```python
from build123d import *

# Parameters (mm, degrees)
F0_W     = 33
F0_H     = 70
F0_W_2   = 12.5
F0_H_2   = 29.0257008746
F0_R     = 1.95
F0_H_3   = 10
F1_DEPTH = 10
F2_DEPTH = 28
F3_START = 10
F3_DEPTH = 11
F4_SIZE2 = 8
F4_SIZE  = 2
F5_R     = 4
F6_R     = 5
F7_R     = 2
F8_R     = 2


with BuildPart() as f1:
    # F0 (on Top) → F1 (new body)
    with BuildSketch(Plane.XY):
        with Locations((-48.7103275061, 13.0742679536)):
            Rectangle(F0_W, F0_H)
        with Locations((-48.9603275061, -3.1253187917)):
            Rectangle(F0_W_2, F0_H_2, mode=Mode.SUBTRACT)
        with Locations((-55.2103275061, 20.0742679536)):
            Circle(F0_R, mode=Mode.SUBTRACT)
        with Locations((-55.2103275061, 32.5742679536)):
            Circle(F0_R, mode=Mode.SUBTRACT)
        with Locations((-42.7103275061, 20.0742679536)):
            Circle(F0_R, mode=Mode.SUBTRACT)
        with Locations((-42.7103275061, 32.5742679536)):
            Circle(F0_R, mode=Mode.SUBTRACT)
        with Locations((-48.7103275061, -26.9257320464)):
            Rectangle(F0_W, F0_H_3)
        with Locations((-48.7103275061, -36.9257320464)):
            Rectangle(F0_W, F0_H_3)
    extrude(amount=F1_DEPTH)

    # F0 (on Top) → F2 (join)
    with BuildSketch(Plane.XY):
        with Locations((-48.7103275061, -26.9257320464)):
            Rectangle(F0_W, F0_H_3)
        with Locations((-48.7103275061, -36.9257320464)):
            Rectangle(F0_W, F0_H_3)
    extrude(amount=F2_DEPTH)

    # F0 (on Top) → F3 (cut)
    with BuildSketch(Plane.XY.offset(F3_START)):
        with Locations((-48.7103275061, -26.9257320464)):
            Rectangle(F0_W, F0_H_3)
    extrude(amount=F3_DEPTH, mode=Mode.SUBTRACT)

    # F4
    f4_edges = [f1.edges().sort_by_distance(p)[0] for p in [
        (-48.710328, -31.925732, 10),
    ]]
    f4_side = f1.faces().sort_by_distance((-33.075718, 8.074268, 10))[0]
    chamfer(f4_edges, length=F4_SIZE, length2=F4_SIZE2, reference=f4_side)

    # F5
    f5_edges = [f1.edges().sort_by_distance(p)[0] for p in [
        (-48.710328, -21.925732, 28),
        (-48.710328, -41.925732, 28),
    ]]
    fillet(f5_edges, radius=F5_R)

    # F6
    f6_edges = [f1.edges().sort_by_distance(p)[0] for p in [
        (-65.210328, 48.074268, 5),
        (-32.210328, 48.074268, 5),
    ]]
    fillet(f6_edges, radius=F6_R)

    # F7
    f7_edges = [f1.edges().sort_by_distance(p)[0] for p in [
        (-42.710328, 11.387532, 5),
        (-55.210328, 11.387532, 5),
        (-55.210328, -17.638169, 5),
        (-42.710328, -17.638169, 5),
    ]]
    fillet(f7_edges, radius=F7_R)

    # F8
    f8_edges = [f1.edges().sort_by_distance(p)[0] for p in [
        (-65.210328, -31.925732, 28),
        (-32.210328, -31.925732, 28),
    ]]
    fillet(f8_edges, radius=F8_R)


solid = f1.part
```
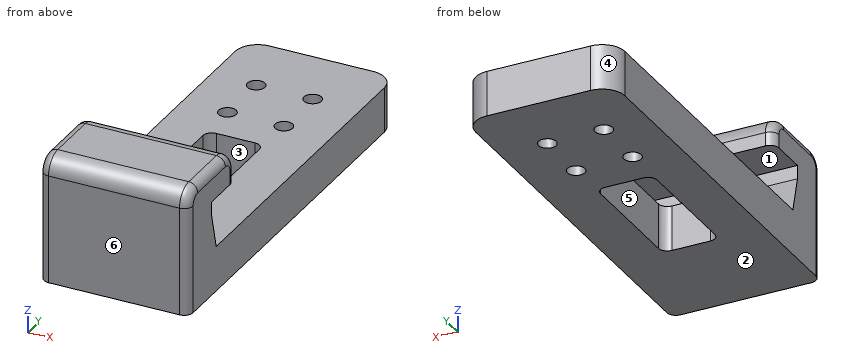
For this review, take the finished solid that the model builds, in its own axes (mm). Face numbers are marked on the shaded views. A direction names the side the tool comes from. Give positions to 0.01 mm unless a question says otherwise; leave off trailing zeros. Order: outer loops, then holes, each group sorted by start corner. A loop starts at its lowest first (then second) coordinate and runs counter-clockwise, first axis right, second up.
1) Insertion check: pin 1 (16.5 mm diameter, centred on x = -49.5, y = -0.5, fed in from +Z); pin 2 (0.9 mm diameter, centred on x = -48.5, z = 19, fed in from +Y); pin 3 (5 mm diameter, centred on y = -20.5, z = 23.5, fed in from -X). Each pin has a flat end and moves straight along its axis. Give the tip position at first contact, or say it passes through.
2) Take a section at C-C (z = 7). Give the boundary of the cut face in (x, y), then the cut area to 3 significant figures.
3) The part is to be moulded in two halves that separate along Y. For the marked faces 4, 5 and 6, say which applies: released by +Y, released by -Y, zero draft, split by the parting line, or undercut.
4) Take a section at D-D (y = -16.5). Give the boundary of the cut face in (x, z).
5) For the marked faces 1, 2 and 3, list the 3-axis set-ups (+Z, -Z, +X, -X, +Y, -Y) from which the entire face can be reached by the end or side of a thin tool; tool diameter is ignored.
6) Wall thickness on line 1 (Y direction, x = -50, z = 1.75); line 2 (Z direction, x = -43.5, y = -26); line 3 (Y direction, x = -41.5, z = 4.75): over which ranges is each line inside the solid? List them lowest first.
7) Take a section at A-A (y = -1.5). Give the boundary of the cut face in (x, z).
8) Take a section at B-B (x = -39.5). Give the boundary of the cut face in (y, z), then the cut area to 3 significant figures.
Derived:
1. pin 1: stops at z = 10
1. pin 2: stops at y = -31.93
1. pin 3: stops at x = -64.98
2. outline: (-65.21, -39.93) arc R2 ccw to (-63.21, -41.93) - (-34.21, -41.93) arc R2 ccw to (-32.21, -39.93) - (-32.21, 43.07) arc R5 ccw to (-37.21, 48.07) - (-60.21, 48.07) arc R5 ccw to (-65.21, 43.07) - close; hole circle Ø3.9 at (-55.21, 20.07); hole circle Ø3.9 at (-55.21, 32.57); hole (-55.21, -15.64) arc R2 ccw to (-53.21, -17.64) - (-44.71, -17.64) arc R2 ccw to (-42.71, -15.64) - (-42.71, 9.39) arc R2 ccw to (-44.71, 11.39) - (-53.21, 11.39) arc R2 ccw to (-55.21, 9.39) - close; hole circle Ø3.9 at (-42.71, 20.07); hole circle Ø3.9 at (-42.71, 32.57)
2. area: 2,550 mm2
3. face 4: released by +Y
3. face 5: undercut
3. face 6: released by -Y
4. outline: (-65.21, 0) - (-55.02, 0) - (-55.02, 10) - (-65.21, 10) - close; (-42.91, 0) - (-32.21, 0) - (-32.21, 10) - (-42.91, 10) - close
5. face 1: +X, -X, +Y
5. face 2: -Z, +X, -X, +Y, -Y
5. face 3: +Z, -Z
6. line 1: y = -41.93 to -17.64, 11.39 to 48.07
6. line 2: z = 0 to 10, 21 to 28
6. line 3: y = -41.93 to 18.55, 21.6 to 31.05, 34.1 to 48.07
7. outline: (-65.21, 0) - (-55.21, 0) - (-55.21, 10) - (-65.21, 10) - close; (-42.71, 0) - (-32.21, 0) - (-32.21, 10) - (-42.71, 10) - close
8. outline: (-41.93, 0) - (48.07, 0) - (48.07, 10) - (-29.93, 10) - (-31.93, 18) - (-31.93, 21) - (-21.93, 21) - (-21.93, 24) arc R4 ccw to (-25.93, 28) - (-37.93, 28) arc R4 ccw to (-41.93, 24) - close
8. area: 1,150 mm2
